from build123d import *

# Parameters (mm, degrees)
SKETCH_1_W      = 12
SKETCH_1_H      = 30
SKETCH_1_R      = 2.65
SKETCH_1_R_2    = 1.25
SKETCH_1_R_3    = 1.75
EXTRUDE_1_DEPTH = 3
FILLET_1_SIZE   = 5
FILLET_1_SIZE_2 = 15
FILLET_2_SIZE   = 5
FILLET_2_SIZE_2 = 15
FILLET_3_SIZE   = 15
FILLET_3_SIZE_2 = 5
FILLET_4_SIZE   = 5
FILLET_4_SIZE_2 = 15


with BuildPart() as part:
    # 草图1 → 凸台-拉伸1 (new body)
    with BuildSketch(Plane.XY):
        with Locations((-4.763664969, 12.565714772)):
            Rectangle(SKETCH_1_W, SKETCH_1_H)
        with Locations((-4.763664969, 12.565714772)):
            Circle(SKETCH_1_R, mode=Mode.SUBTRACT)
        with Locations((-4.763664969, 23.875723392)):
            Circle(SKETCH_1_R_2, mode=Mode.SUBTRACT)
        with Locations((-4.763664969, 18.875154811)):
            Circle(SKETCH_1_R_3, mode=Mode.SUBTRACT)
        with Locations(Location((-4.763664969, 1.255706152, 0), (0, 0, 180))):
            Circle(SKETCH_1_R_2, mode=Mode.SUBTRACT)
        with Locations(Location((-4.763664969, 6.256274734, 0), (0, 0, 180))):
            Circle(SKETCH_1_R_3, mode=Mode.SUBTRACT)
    extrude(amount=EXTRUDE_1_DEPTH)

    # 圆角1
    # an asymmetric fillet: 15, 5 mm, written as the material it takes off along each edge
    with BuildSketch(Plane(origin=(-10.763664969, 27.565714772, -37.5), x_dir=(1, 0, 0), z_dir=(0, 0, 1))) as fillet_1_piece_1:
        with BuildLine():
            Bezier((FILLET_1_SIZE, 0), (0, 0), (0, -FILLET_1_SIZE_2), weights=[1, 0.707106781, 1])
            Line((0, -FILLET_1_SIZE_2), (0, 0))
            Line((0, 0), (FILLET_1_SIZE, 0))
        make_face()
    extrude(amount=78, mode=Mode.SUBTRACT)

    # 圆角2
    # an asymmetric fillet: 15, 5 mm, written as the material it takes off along each edge
    with BuildSketch(Plane(origin=(1.236335031, 27.565714772, -37.5), x_dir=(-1, 0, 0), z_dir=(0, 0, 1))) as fillet_2_piece_1:
        with BuildLine():
            Bezier((FILLET_2_SIZE, 0), (0, 0), (0, FILLET_2_SIZE_2), weights=[1, 0.707106781, 1])
            Line((0, FILLET_2_SIZE_2), (0, 0))
            Line((0, 0), (FILLET_2_SIZE, 0))
        make_face()
    extrude(amount=78, mode=Mode.SUBTRACT)

    # 圆角3
    # an asymmetric fillet: 15, 5 mm, written as the material it takes off along each edge
    with BuildSketch(Plane(origin=(-10.763664969, -2.434285228, -37.5), x_dir=(0, 1, 0), z_dir=(0, 0, 1))) as fillet_3_piece_1:
        with BuildLine():
            Bezier((FILLET_3_SIZE, 0), (0, 0), (0, -FILLET_3_SIZE_2), weights=[1, 0.707106781, 1])
            Line((0, -FILLET_3_SIZE_2), (0, 0))
            Line((0, 0), (FILLET_3_SIZE, 0))
        make_face()
    extrude(amount=78, mode=Mode.SUBTRACT)

    # 圆角4
    # an asymmetric fillet: 15, 5 mm, written as the material it takes off along each edge
    with BuildSketch(Plane(origin=(1.236335031, -2.434285228, -37.5), x_dir=(-1, 0, 0), z_dir=(0, 0, 1))) as fillet_4_piece_1:
        with BuildLine():
            Bezier((FILLET_4_SIZE, 0), (0, 0), (0, -FILLET_4_SIZE_2), weights=[1, 0.707106781, 1])
            Line((0, -FILLET_4_SIZE_2), (0, 0))
            Line((0, 0), (FILLET_4_SIZE, 0))
        make_face()
    extrude(amount=78, mode=Mode.SUBTRACT)


solid = part.part
Input: part model. Units: mm. Frame: model coordinates. Coordinates: 2 decimals unless noted, no trailing zeros. Write each loop counter-clockwise with the first axis right and the second up, starting at its lowest first coordinate (ties: lowest second). Pieces come first, ordered by that corner, then holes. Notation, with made-up numbers: M 56,29.25 L 108,29.25 A12 cw 108,40.25 Z; hole C 4,-26.75 d5. An arc over 180 degrees is marked long. Answer as a JSON object with one key per item and string values. Group by question number.
(1) Contact query for flat-ended pins moving along their axis: P1, Ø2, axis at x = -4.76, y = 6.26, coming from the +Z side; P2, Ø1.5, axis at y = 19.5, z = 0.5, coming from the +X side. Output: stop coordinate, or through.
(2) Ray query, line 1 along Y through (x, z) = (-4.75, 0.85); line 2 along Y through (x, z) = (-4.5, 2.6); line 3 along X through (y, z) = (6.5, 2.8). Return the intervals inside material, ascending. Write a range as [from, to].
(3) Section B-B on z = 2.5. Give the number of separate pieces and of enclosed holes in the cut face, plus the area to 3 significant figures.
(4) Section A-A on x = -4.25. Output: boundary loops of the cut face in (y, z).
(5) Mould query, pull axis X, two halves, no side actions, for faces 1 (the face through (-5, 27.566, 1)), 2 (the face through (-3.515, 1.201, 1.479)). Classes: pulls with the +X half, pulls with the -X half, needs draft (parallel to the pull), parting line crosses it, or undercut.
Result set:
{
 "1": {"P1": "passes through", "P2": "stops at x = 0.79"},
 "2": {"line 1": "y = [-2.43, 0.01], [2.51, 4.51], [8.01, 9.92], [15.22, 17.13], [20.63, 22.63], [25.13, 27.57]", "line 2": "y = [-2.43, 0.03], [2.48, 4.53], [7.99, 9.93], [15.2, 17.15], [20.61, 22.65], [25.1, 27.57]", "line 3": "x = [-10.34, -6.5], [-3.03, 0.81]"},
 "3": {"separate pieces": "1", "enclosed holes": "5", "area": "244 mm2"},
 "4": {"outline": "M -2.43,0 L 0.12,0 L 0.12,3 L -2.43,3 Z; M 2.4,0 L 4.58,0 L 4.58,3 L 2.4,3 Z; M 7.93,0 L 9.97,0 L 9.97,3 L 7.93,3 Z; M 15.17,0 L 17.2,0 L 17.2,3 L 15.17,3 Z; M 20.55,0 L 22.74,0 L 22.74,3 L 20.55,3 Z; M 25.02,0 L 27.57,0 L 27.57,3 L 25.02,3 Z"},
 "5": {"face 1": "needs draft", "face 2": "undercut"}
}
